Model file for the job. Use its own axes, mm. Face numbers are marked on the shaded views. A direction names the side the tool comes from. Give positions to 0.01 mm unless a question says otherwise; leave off trailing zeros. Loops run counter-clockwise (first coordinate to the right, second up) from the corner with the lowest first, then second, coordinate; pieces in that order, holes last. Notation, with made-up numbers: M 37,-6.5 L 80,-6.5 A29 ccw 80,22.5 Z; hole C 10.5,24 d2. An arc over 180 degrees is marked long. Answer in a Markdown table with one row per item.
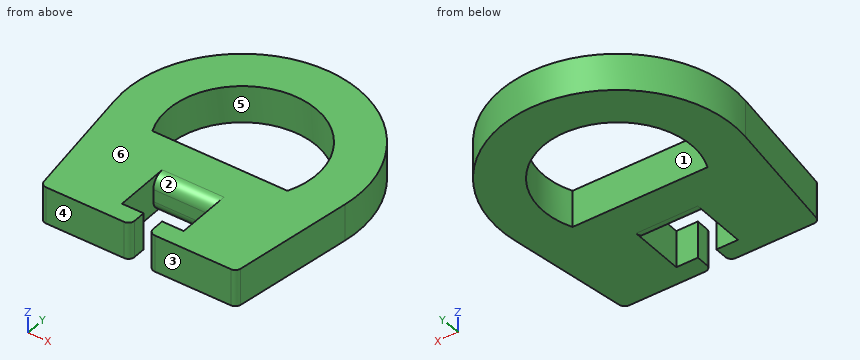
```python
from build123d import *

# Parameters (mm, degrees)
F1_DEPTH = 3
F2_R     = 1


with BuildPart() as f1:
    # F0 (on Top) → F1 (new body)
    with BuildSketch(Plane.XY):
        with BuildLine():
            Line((-28.706517, 10.57433), (-28.706517, 14.07433))
            Line((-28.706517, 14.07433), (-23.706517, 14.07433))
            Line((-23.706517, 14.07433), (-23.706517, 10.57433))
            Line((-23.706517, 10.57433), (-25.456517, 10.57433))
            Line((-25.456517, 10.57433), (-25.456517, 9.57433))
            ThreePointArc((-25.456517, 9.57433), (-25.31007, 9.220777), (-24.956517, 9.07433))
            Line((-24.956517, 9.07433), (-23.706517, 9.07433))
            Line((-23.706517, 9.07433), (-22.618948, 9.07433))
            Line((-22.618948, 9.07433), (-18.791793, 9.07433))
            ThreePointArc((-18.791793, 9.07433), (-18.466205, 9.194866), (-18.297598, 9.498359))
            Line((-18.297598, 9.498359), (-16.816818, 19.130878))
            ThreePointArc((-16.816818, 19.130878), (-26.134756, 30.074059), (-35.61695, 19.272893))
            Line((-35.61695, 19.272893), (-34.266192, 9.505833))
            ThreePointArc((-34.266192, 9.505833), (-34.099351, 9.197336), (-33.770906, 9.07433))
            Line((-33.770906, 9.07433), (-29.794085, 9.07433))
            Line((-29.794085, 9.07433), (-27.456517, 9.07433))
            ThreePointArc((-27.456517, 9.07433), (-27.102963, 9.220777), (-26.956517, 9.57433))
            Line((-26.956517, 9.57433), (-26.956517, 10.57433))
            Line((-26.956517, 10.57433), (-28.706517, 10.57433))
        make_face()
        with BuildLine():
            Line((-20.729291, 18.07433), (-31.683742, 18.07433))
            ThreePointArc((-31.683742, 18.07433), (-26.206517, 26.595127), (-20.729291, 18.07433))
        make_face(mode=Mode.SUBTRACT)
    extrude(amount=F1_DEPTH)

    # F2
    f2_edges = [f1.edges().sort_by_distance(p)[0] for p in [
        (-26.206517, 14.07433, 3),
        (-26.206517, 14.07433, 0),
    ]]
    fillet(f2_edges, radius=F2_R)


solid = f1.part
```
(1) Saw through at C-C, the plane z = 0.3. Give the cut face in (x, y).
Established:
| item | result |
|---|---|
| outline | M -35.62,19.27 L -34.27,9.51 A0.5 ccw -33.77,9.07 L -27.46,9.07 A0.5 ccw -26.96,9.57 L -26.96,10.57 L -28.71,10.57 L -28.71,14.36 L -23.71,14.36 L -23.71,10.57 L -25.46,10.57 L -25.46,9.57 A0.5 ccw -24.96,9.07 L -18.79,9.07 A0.5 ccw -18.3,9.5 L -16.82,19.13 A9.5 ccw long Z; hole M -31.68,18.07 L -20.73,18.07 A6.02 ccw long Z |
(2) Saw through at A-A, the plane y = 13.5. Give the cut face in (x, z), and give its area (3 significant figures).
Established:
| item | result |
|---|---|
| outline | M -34.82,0 L -28.71,0 L -28.71,3 L -34.82,3 Z; M -23.71,0 L -17.68,0 L -17.68,3 L -23.71,3 Z |
| area | 36.4 mm2 |
(3) Wall check: L1, parallel to Y at x = -26.25, z = 2; L2, parallel to Y at x = -25, z = 2; L3, parallel to X at y = 20.75, z = 0.65. Give the ranges that are in metal, low to high.
Established:
| item | result |
|---|---|
| L1 | y = 14.07 to 18.07, 26.59 to 30.07 |
| L2 | y = 9.08 to 10.57, 14.07 to 18.07, 26.47 to 30 |
| L3 | x = -35.7 to -32.22, -20.19 to -16.71 |
(4) Flat gauge pins, fed straight in: P1, Ø0.9, axis at x = -27.5, z = 1, coming from the +Y side; P2, Ø0.8, axis at y = 10, z = 1, coming from the +X side; P3, Ø1.5, axis at y = 13.5, z = 2, coming from the +X side. Where does each tip first touch, or does it go through?
Established:
| item | result |
|---|---|
| P1 | stops at y = 30.04 |
| P2 | stops at x = -18.16 |
| P3 | stops at x = -17.57 |
(5) Saw through at B-B, the plane x = -26.5. Give the cut face in (y, z).
Established:
| item | result |
|---|---|
| outline | M 14.07,1 A1 ccw 15.07,0 L 18.07,0 L 18.07,3 L 15.07,3 A1 ccw 14.07,2 Z; M 26.59,0 L 30.07,0 L 30.07,3 L 26.59,3 Z |
(6) Which spindle directions (+Z, -Z, +X, -X, +Y, -Y) get a long thin tool onto all of the face, cutting with end or side? Do the marked faces 1, 2 and 3. Say none if no direction does.
Established:
| item | result |
|---|---|
| face 1 | +Z, -Z |
| face 2 | +Z |
| face 3 | +Z, -Z, +X, -X, -Y |
(7) Saw through at D-D, the plane y = 19.75. Give the cut face in (x, z), and give its area (3 significant figures).
Established:
| item | result |
|---|---|
| outline | M -35.67,0 L -32.17,0 L -32.17,3 L -35.67,3 Z; M -20.24,0 L -16.74,0 L -16.74,3 L -20.24,3 Z |
| area | 21.0 mm2 |
(8) Mould opens along Y. For the marked faces 4, 5 and 6 say: pulls with the +Y half, pulls with the -Y half, needs draft (parallel to the pull), parting line crosses it, or undercut.
Established:
| item | result |
|---|---|
| face 4 | pulls with the -Y half |
| face 5 | undercut |
| face 6 | needs draft |
